from build123d import *

# Parameters (mm, degrees)
SKIZZE1_R                       = 52.5
SKIZZE1_R_2                     = 30
AUFSATZ_LINEAR_AUSTRAGEN1_DEPTH = 20
AUFSATZ_LINEAR_START            = 10
SKIZZE2_R                       = 52.5
SKIZZE2_R_2                     = 5
AUFSATZ_LINEAR_AUSTRAGEN2_DEPTH = 10
SKIZZE3_W                       = 9
SKIZZE3_H                       = 14.2
AUFSATZ_LINEAR_AUSTRAGEN3_DEPTH = 19


with BuildPart() as part:
    # Skizze1 → Aufsatz-Linear austragen1 (new body)
    with BuildSketch(Plane(origin=(0, 0, 0), x_dir=(1, 0, 0), z_dir=(0, 1, 0))):
        with Locations(Location((0, 0, 0), (0, 0, 270))):
            Circle(SKIZZE1_R)
        with Locations(Location((0, 0, 0), (0, 0, 270))):
            Circle(SKIZZE1_R_2, mode=Mode.SUBTRACT)
    extrude(amount=AUFSATZ_LINEAR_AUSTRAGEN1_DEPTH)

    # Skizze2 → Aufsatz-Linear austragen2 (add)
    with BuildSketch(Plane.XZ.offset(AUFSATZ_LINEAR_START)):
        with Locations(Location((0, 0, 0), (0, 0, 270))):
            Circle(SKIZZE2_R)
        with Locations(Location((0, 0, 0), (0, 0, 270))):
            Circle(SKIZZE2_R_2, mode=Mode.SUBTRACT)
    extrude(amount=-AUFSATZ_LINEAR_AUSTRAGEN2_DEPTH)

    # Skizze3 → Aufsatz-Linear austragen3 (add)
    with BuildSketch(Plane(origin=(0, 20, 0), x_dir=(1, 0, 0), z_dir=(0, 1, 0))):
        with Locations((0, -36.7605799)):
            Rectangle(SKIZZE3_W, SKIZZE3_H)
    extrude(amount=AUFSATZ_LINEAR_AUSTRAGEN3_DEPTH)


solid = part.part
Check sheet for the modelled part. Datum: model origin and axes. Units: mm. A direction names the side the tool comes from. Coordinates: 2 decimals unless noted, no trailing zeros. Write each loop counter-clockwise with the first axis right and the second up, starting at its lowest first coordinate (ties: lowest second). Pieces come first, ordered by that corner, then holes.
Item 1: Mould release check, pull along Z, two halves, no side actions. Record for faces 4 (the face through (-4.88, -5.07, 1.08)), 5 (the face through (0, 39, 37)), 6 (the face through (0, 29, 43.861)): released by +Z, released by -Z, zero draft, split by the parting line, or undercut.
Numbers:
face 4: undercut
face 5: zero draft
face 6: released by +Z
Item 2: Scan lines: probe 1 along X at (y, z) = (9.75, 0); probe 2 along X at (y, z) = (-6, 0); probe 3 along Y at (x, z) = (15.5, 43). Record each from-to range of solid material in increasing order.
Numbers:
probe 1: x = -52.5 to -30, 30 to 52.5
probe 2: x = -52.5 to -5, 5 to 52.5
probe 3: y = -10 to 20
Item 3: Cross-section at B-B on z = 0. Record the boundary of the cut face in (x, y).
Numbers:
outline: (-52.5, -10) - (-5, -10) - (-5, 0) - (-30, 0) - (-30, 20) - (-52.5, 20) - close; (5, -10) - (52.5, -10) - (52.5, 20) - (30, 20) - (30, 0) - (5, 0) - close
Item 4: Cross-section at C-C on z = 31.5. Record the boundary of the cut face in (x, y).
Numbers:
outline: (-42, -10) - (42, -10) - (42, 20) - (4.5, 20) - (4.5, 39) - (-4.5, 39) - (-4.5, 20) - (-42, 20) - close
Item 5: Cross-section at D-D on y = -6.5. Record the boundary of the cut face in (x, z), then the cut area to 3 significant figures.
Numbers:
outline: circle Ø105 at (0, 0); hole circle Ø10 at (0, 0)
area: 8,580 mm2
Item 6: Cross-section at A-A on x = 0. Record the boundary of the cut face in (y, z).
Numbers:
outline: (-10, -52.5) - (20, -52.5) - (20, -30) - (0, -30) - (0, -5) - (-10, -5) - close; (-10, 5) - (0, 5) - (0, 30) - (20, 30) - (20, 29.66) - (39, 29.66) - (39, 43.86) - (20, 43.86) - (20, 52.5) - (-10, 52.5) - close
Item 7: Depth check by flat-ended pin: pin 1 Ø4 at (x, y) = (32.5, 6) entering from -Z; pin 2 Ø1 at (x, y) = (-34.5, -3.5) entering from -Z; pin 3 Ø4 at (x, y) = (41, 15) entering from +Z. Enter the tip coordinate at first touch or a pass-through.
Numbers:
pin 1: stops at z = -42.73
pin 2: stops at z = -40
pin 3: stops at z = 35.15
Item 8: Access from +Z, -Z, +X, -X, +Y, -Y to the whole of each face (thin tool, end or side, straight path). Record for faces 1 (the face through (-4.5, 29, 37)), 2 (the face through (4.5, 29, 37)), 3 (the face through (0, 29, 29.661)).
Numbers:
face 1: +Z, -Z, -X, +Y
face 2: +Z, -Z, +X, +Y
face 3: -Z, +X, -X, +Y
